Drawing for the job (mm, zero at the part's lowest x, y, z). Give positions to 0.01 mm unless a question says otherwise; leave off trailing zeros. Loops run counter-clockwise (first coordinate to the right, second up) from the corner with the lowest first, then second, coordinate; pieces in that order, holes last. Notation, with made-up numbers: M 60,-6.75 L 87,-6.75 A27 ccw 87,13.25 Z; hole C -18.75,73 d9. An arc over 180 degrees is marked long. Answer in a Markdown table with one row per item. Add a question column.
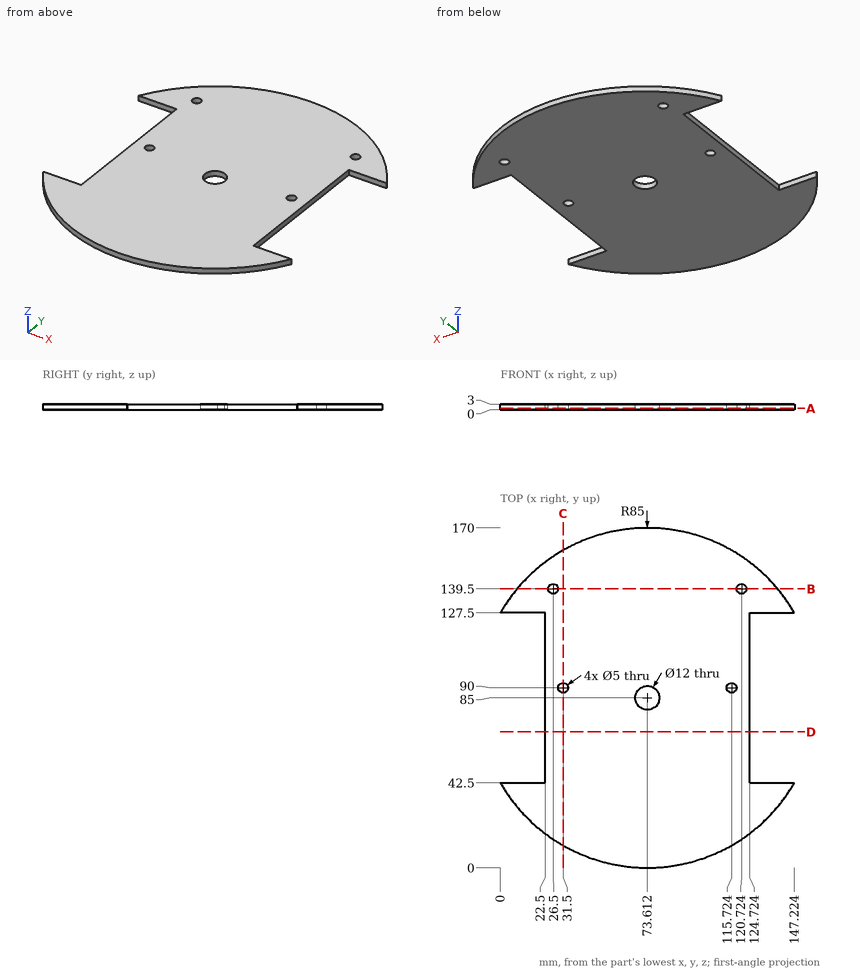
(1) Wall check: line 1 (X direction, y = 139.5, z = 2.3) (1 decimal); line 2 (Y direction, x = 122.5, z = 0.65) (1 decimal); line 3 (Y direction, x = 136, z = 2.5). Give the ranges that are in metal, low to high.
(2) Slice it at A-A, the plane z = 0.85. Give the cut face in (x, y), then the cut area to 3 significant figures.
(3) Pin check, flat tips, straight feed: pin 1 (1 mm diameter, centred on y = 52, z = 0.5, fed in from +X); pin 2 (1.5 mm diameter, centred on y = 76, z = 2, fed in from -X); pin 3 (4 mm diameter, centred on x = 31.5, y = 90, fed in from +Z); pin 4 (1 mm diameter, centred on x = 57, z = 1, fed in from -Y). Stop position of each tip, or through.
(4) Slice it at C-C, the plane x = 31.5. Give the cut face in (y, z) (1 decimal).
(5) Slice it at B-B, the plane y = 139.5. Give the cut face in (x, z).
(6) Slice it at D-D, the plane y = 68. Give the cut face in (x, z), then the cut area to 3 significant figures.
Solution:
| question | item | result |
|---|---|---|
| 1 | line 1 | 8.4 to 24, 29 to 118.2, 123.2 to 138.8 |
| 1 | line 2 | 15.5 to 137.7, 141.3 to 154.5 |
| 1 | line 3 | 27.27 to 42.5, 127.5 to 142.73 |
| 2 | outline | M 0,42.5 A85 ccw 147.22,42.5 L 124.72,42.5 L 124.72,127.5 L 147.22,127.5 A85 ccw 0,127.5 L 22.5,127.5 L 22.5,42.5 Z; hole C 26.5,139.5 d5; hole C 31.5,90 d5; hole C 73.61,85 d12; hole C 115.72,90 d5; hole C 120.72,139.5 d5 |
| 2 | area | 17,400 mm^2 |
| 3 | pin 1 | x = 124.72 |
| 3 | pin 2 | x = 22.5 |
| 3 | pin 3 | through |
| 3 | pin 4 | y = 1.54 |
| 4 | outline | M 11.2,0 L 87.5,0 L 87.5,3 L 11.2,3 Z; M 92.5,0 L 158.8,0 L 158.8,3 L 92.5,3 Z |
| 5 | outline | M 8.38,0 L 24,0 L 24,3 L 8.38,3 Z; M 29,0 L 118.22,0 L 118.22,3 L 29,3 Z; M 123.22,0 L 138.84,0 L 138.84,3 L 123.22,3 Z |
| 6 | outline | M 22.5,0 L 124.72,0 L 124.72,3 L 22.5,3 Z |
| 6 | area | 307 mm^2 |
